Check sheet for the modelled part. Datum: model origin and axes. Units: mm. Face numbers are marked on the shaded views. A direction names the side the tool comes from. Give positions to 0.01 mm unless a question says otherwise; leave off trailing zeros. Loops run counter-clockwise (first coordinate to the right, second up) from the corner with the lowest first, then second, coordinate; pieces in that order, holes last. Notation, with made-up numbers: M 52.25,-36.75 L 100.25,-36.75 A20 cw 100.25,-3.75 Z; hole C 2,45 d4. An arc over 180 degrees is marked long. Put each result on its own line as item: value. Start each with the question number.
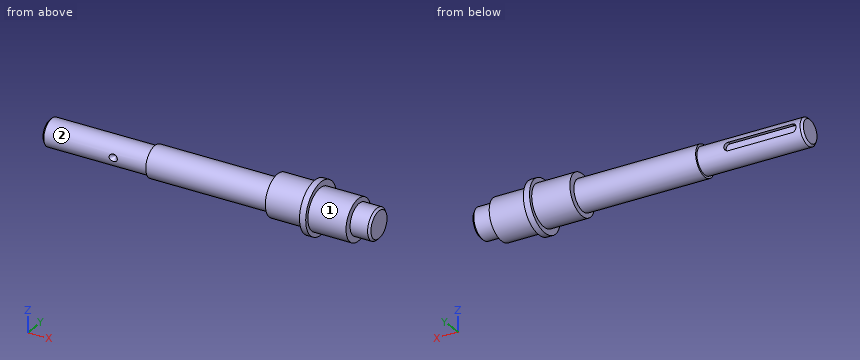
```python
from build123d import *

# Parameters (mm, degrees)
CUT_EXTRUDE_START   = 13
CUT_EXTRUDE_1_DEPTH = 4
SKETCH_3_R          = 20
EXTRUDE_1_DEPTH     = 37
SKETCH_4_R          = 20
EXTRUDE_2_DEPTH     = 37
CHAMFER_1_SIZE      = 2


with BuildPart() as part:
    # 草图1 → 旋转1 (revolve)
    with BuildSketch(Plane.XY, mode=Mode.PRIVATE) as revolve_1_sk:
        Polygon((0, 0), (0, 13), (102, 13), (102, 15), (220, 15), (257, 15), (257, 25), (263, 25), (263, 15), (300, 15), (319, 15), (319, 0), align=None)
    revolve(revolve_1_sk.sketch.rotate(Axis((0, 0, 0), (1, 0, 0)), 90), axis=Axis((0, 0, 0), (1, 0, 0)))

    # 草图2 → 切除-拉伸1 (cut)
    with BuildSketch(Plane(origin=(0, 0, 0), x_dir=(1, 0, 0), z_dir=(0, 1, 0)).offset(CUT_EXTRUDE_START)):
        with BuildLine():
            Line((10, 4), (72, 4))
            ThreePointArc((72, 4), (76, 0), (72, -4))
            Line((72, -4), (10, -4))
            ThreePointArc((10, -4), (6, 0), (10, 4))
        make_face()
    extrude(amount=-CUT_EXTRUDE_1_DEPTH, mode=Mode.SUBTRACT)

    # 草图3 → 凸台-拉伸1 (add)
    with BuildSketch(Plane.ZY.offset(-257)):
        with Locations(Location((0, 1.5, 0), (0, 0, 180))):
            Circle(SKETCH_3_R)
    extrude(amount=EXTRUDE_1_DEPTH)

    # 草图4 → 凸台-拉伸2 (add)
    with BuildSketch(Plane(origin=(263, 0, 0), x_dir=(0, 0, -1), z_dir=(1, 0, 0))):
        with Locations(Location((0, -1.5, 0), (0, 0, 180))):
            Circle(SKETCH_4_R)
    extrude(amount=EXTRUDE_2_DEPTH)

    # 倒角1
    chamfer_1_edges = [part.edges().sort_by_distance(p)[0] for p in [
        (0, 0, -13),
        (319, 0, -15),
    ]]
    chamfer(chamfer_1_edges, length=CHAMFER_1_SIZE)

    # 草图5 → 切除-旋转1 (revolve, cut)
    with BuildSketch(Plane.XY, mode=Mode.PRIVATE) as cut_revolve_1_sk:
        Polygon((65.25, -13), (69.25, -9), (69.25, -13), align=None)
    revolve(cut_revolve_1_sk.sketch.rotate(Axis((69.25, -17.970703126, 0), (0, 1, 0)), 270), axis=Axis((69.25, -17.970703126, 0), (0, 1, 0)), mode=Mode.SUBTRACT)


solid = part.part
```
Q1. Depth check by flat-ended pin: P1, Ø1, axis at x = 48.5, y = 10, coming from the +Z side; P2, Ø1, axis at x = 55.5, y = 10.5, coming from the -Z side; P3, Ø6, axis at x = 233, y = 2, coming from the +Z side. Enter the tip coordinate at first touch or a pass-through.
Q2. Section check B-B, the plane x = 113.5. Record the cut outline in (y, z).
Q3. Thickness scan on line 1 along Y through (x, z) = (14, 0); line 2 along X through (y, z) = (13, 21); line 3 along X through (y, z) = (-2, -19.5). Record the ranges inside material, lowest first. Write a range as [from, to].
Q4. Access from +Z, -Z, +X, -X, +Y, -Y to the whole of each face (thin tool, end or side, straight path). Record for the marked faces 1 and 2.
Q5. Section check A-A, the plane x = 270.5. Record the cut outline in (y, z), then the cut area to 3 significant figures.
Found:
1. P1: stops at z = 8.87
1. P2: stops at z = -8.31
1. P3: stops at z = 20
2. outline: C 0,0 d30
3. line 1: y = [-13, 9]
3. line 2: x = [257, 263]
3. line 3: x = [220, 300]
4. face 1: +X
4. face 2: -X
5. outline: C -1.5,0 d40
5. area: 1,260 mm^2
